Can you work these out from the model? Positions are in its coordinate system, mm. Face numbers are marked on the shaded views. A direction names the side the tool comes from. Coordinates: 2 decimals unless noted, no trailing zeros. Order: outer loops, then holes, each group sorted by start corner. A loop starts at its lowest first (then second) coordinate and runs counter-clockwise, first axis right, second up. Notation, with made-up numbers: (12.5, 52) -> (26.5, 52) arc R6 ccw to (26.5, 61) -> close; hole circle Ø11 at (15, 83.5). An arc over 180 degrees is marked (long way). Use a Markdown table: item, result. Add a question column.
1. Suppose I cut it at B-B, the plane z = 8. List the corners of the cut face in (x, y) for me, then the cut area to 3 significant figures.
2. If I drill on line 1 along Y through (x, z) = (0, 10); line 2 along Z through (x, y) = (6.75, 7.5); line 3 along Y through (x, z) = (0, -3), over which ranges is the centre line in solid material (lowest first)? Write a range as from..to.
3. Suppose I cut it at A-A, the plane y = -2. List the corners of the cut face in (x, z) for me, then the cut area to 3 significant figures.
4. For pin 1 Ø12 at (x, y) = (7.5, 8.5) entering from -Z; pin 2 Ø4 at (x, y) = (-1.5, -1) entering from -Z; pin 3 Ø4 at (y, z) = (-3.5, 15.5) entering from +X; pin 4 Ø5 at (x, z) = (-3, 11.5) entering from +Y, each with a flat end and sliding along its axis, tell me the tip position at first contact or that it passes through.
5. We'd pull the mould along Z, two halves only. Please class the marked faces 4, 5 and 6: pulls with the +Z half, pulls with the -Z half, needs draft (parallel to the pull), parting line crosses it, or undercut.
6. Suppose I cut it at C-C, the plane y = -4.5. List the corners of the cut face in (x, z) for me.
7. Suppose I cut it at D-D, the plane x = 18. List the corners of the cut face in (y, z) for me.
8. For the marked faces 1, 2 and 3, which set-ups out of +Z, -Z, +X, -X, +Y, -Y let a thin tool reach every point of the face, with its end or its side?
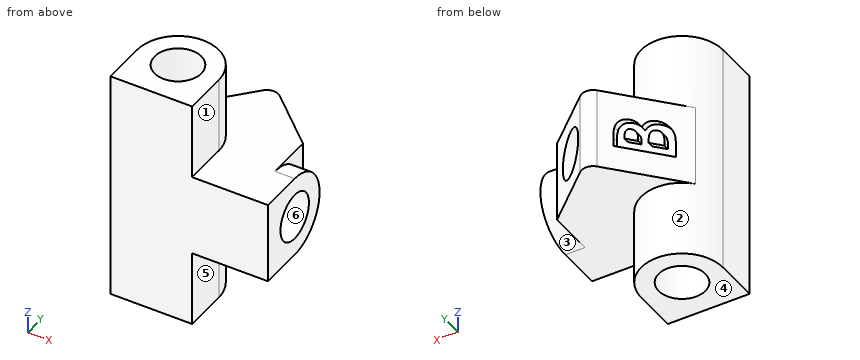
```python
from build123d import *

# Parameters (mm, degrees)
DODANIE_WYCI_GNI_CIE1_DEPTH             = 20
DODANIE_WYCI_GNI_CIE1_DEPTH_BACK        = 20
SZKIC1_R                                = 7
SZKIC1_R_2                              = 4
DODANIE_WYCI_GNI_CIE2_DEPTH             = 10
DODANIE_WYCI_GNI_CIE2_DEPTH_BACK        = 10
SZKIC2_R                                = 4
DODANIE_WYCI_GNI_CIE4_REACH             = 28.181
DODANIE_WYCI_GNI_CIE4_END_RADIUS        = 7
SZKIC3_W                                = 14
SZKIC3_H                                = 14
DODANIE_WYCI_GNI_CIE4_DIRECTION_2_DEPTH = 10
SZKIC9_R                                = 7
DODANIE_WYCI_GNI_CIE6_DEPTH             = 20
DODANIE_WYCI_GNI_CIE5_REACH             = 39.607
SZKIC12_R                               = 4
WYTNIJ_WYCI_GNI_CIE3_DEPTH              = 40.984557912
DODANIE_WYCI_GNI_CIE7_START             = 8
DODANIE_WYCI_GNI_CIE7_DEPTH             = 8.618630395
SZKIC4_R                                = 4
WYTNIJ_WYCI_GNI_CIE1_DEPTH              = 10
SZKIC10_R                               = 4
WYTNIJ_WYCI_GNI_CIE2_DEPTH              = 10
ZAOKR_GLENIE1_R                         = 2
WYTNIJ_WYCI_GNI_CIE4_DEPTH              = 1


with BuildPart() as part:
    # Szkic1 → Dodanie-wyciągnięcie1 (new, two sides: drawn at the far end of the back side and taken through both)
    with BuildSketch(Plane.XY.offset(-DODANIE_WYCI_GNI_CIE1_DEPTH_BACK)):
        Circle(SZKIC1_R)
        Circle(SZKIC1_R_2, mode=Mode.SUBTRACT)
    extrude(amount=DODANIE_WYCI_GNI_CIE1_DEPTH + DODANIE_WYCI_GNI_CIE1_DEPTH_BACK)

    # Szkic2 → Dodanie-wyciągnięcie2 (add, two sides: drawn at the far end of the back side and taken through both)
    with BuildSketch(Plane.XY.offset(-DODANIE_WYCI_GNI_CIE2_DEPTH_BACK)):
        Circle(SZKIC2_R)
    extrude(amount=DODANIE_WYCI_GNI_CIE2_DEPTH + DODANIE_WYCI_GNI_CIE2_DEPTH_BACK)

    # Dodanie-wyciągnięcie4: up to this cylinder (the profile starts outside it)
    dodanie_wyci_gni_cie4_end = Plane(origin=(0, 0, 0), z_dir=(0, 0, 1)) * Cylinder(DODANIE_WYCI_GNI_CIE4_END_RADIUS, 71.362, mode=Mode.PRIVATE)
    # Szkic3 → Dodanie-wyciągnięcie4 (add, up to the surface)
    with BuildSketch(Plane(origin=(4.711087595, 5.177417665, 0), x_dir=(0, 0, 1), z_dir=(0.6730125135097745, 0.7396310949786087, 0)), mode=Mode.PRIVATE) as dodanie_wyci_gni_cie4_sk1:
        Rectangle(SZKIC3_W, SZKIC3_H)
    dodanie_wyci_gni_cie4_tool1 = extrude(dodanie_wyci_gni_cie4_sk1.sketch, amount=-DODANIE_WYCI_GNI_CIE4_REACH, mode=Mode.PRIVATE) - dodanie_wyci_gni_cie4_end
    add(dodanie_wyci_gni_cie4_tool1.solids().sort_by_distance((4.711088, 5.177418, 0))[0])
    add(dodanie_wyci_gni_cie4_tool1.solids().sort_by_distance((4.711088, 5.177418, 0))[1])

    # Szkic3 → Dodanie-wyciągnięcie4 direction 2 (add)
    with BuildSketch(Plane(origin=(4.711087595, 5.177417665, 0), x_dir=(0, 0, 1), z_dir=(0.6730125135097745, 0.7396310949786087, 0))):
        Rectangle(SZKIC3_W, SZKIC3_H)
    extrude(amount=DODANIE_WYCI_GNI_CIE4_DIRECTION_2_DEPTH)

    # Szkic9 → Dodanie-wyciągnięcie6 (add)
    with BuildSketch(Plane(origin=(0, 0, 0), x_dir=(0, 0, -1), z_dir=(1, 0, 0))):
        Circle(SZKIC9_R)
    extrude(amount=DODANIE_WYCI_GNI_CIE6_DEPTH)

    # Szkic8 → Dodanie-wyciągnięcie5 (add, up to next)
    with BuildSketch(Plane(origin=(0, -7.5, 0), x_dir=(1, 0, 0), z_dir=(0, 1, 0)), mode=Mode.PRIVATE) as dodanie_wyci_gni_cie5_sk1:
        Polygon((7, 20), (-7, 20), (-7, -20), (7, -20), (7, -7), (20, -7), (20, 7), (7, 7), align=None)
    dodanie_wyci_gni_cie5_tool1 = extrude(dodanie_wyci_gni_cie5_sk1.sketch, amount=DODANIE_WYCI_GNI_CIE5_REACH, mode=Mode.PRIVATE) - part.part
    add(dodanie_wyci_gni_cie5_tool1.solids().sort_by_distance((3.311321, -7.5, 0))[0])

    # Szkic12 → Wytnij-wyciągnięcie3 (cut, through all)
    with BuildSketch(Plane.XY.offset(10)):
        Circle(SZKIC12_R)
    extrude(amount=-WYTNIJ_WYCI_GNI_CIE3_DEPTH, mode=Mode.SUBTRACT)

    # Dodanie-wyciągnięcie7: read off the stored shape, not the designer's step
    # Dodanie-wyciągnięcie7 outline → Dodanie-wyciągnięcie7 (add)
    with BuildSketch(Plane.YZ.offset(DODANIE_WYCI_GNI_CIE7_START)):
        with BuildLine():
            Line((7.86264102, 7), (0, 7))
            ThreePointArc((0, 7), (7, 0), (0, -7))
            Line((0, -7), (7.86264102, -7))
            Line((7.86264102, -7), (7.86264102, 7))
        make_face()
    extrude(amount=DODANIE_WYCI_GNI_CIE7_DEPTH)

    # Szkic4 → Wytnij-wyciągnięcie1 (cut)
    with BuildSketch(Plane(origin=(11.44121273, 12.573728615, 0), x_dir=(0, 0, -1), z_dir=(0.6730125135097745, 0.7396310949786088, 0))):
        with Locations(Location((0, 0, 0), (0, 0, 90))):
            Circle(SZKIC4_R)
    extrude(amount=-WYTNIJ_WYCI_GNI_CIE1_DEPTH, mode=Mode.SUBTRACT)

    # Szkic10 → Wytnij-wyciągnięcie2 (cut)
    with BuildSketch(Plane(origin=(20, 0, 0), x_dir=(0, 0, -1), z_dir=(1, 0, 0))):
        Circle(SZKIC10_R)
    extrude(amount=-WYTNIJ_WYCI_GNI_CIE2_DEPTH, mode=Mode.SUBTRACT)

    # Zaokrąglenie1
    zaokr_glenie1_edges = [part.edges().sort_by_distance(p)[0] for p in [
        (6.263795065, 17.284816209, 0),
    ]]
    fillet(zaokr_glenie1_edges, radius=ZAOKR_GLENIE1_R)

    # Szkic14 → Wytnij-wyciągnięcie4 (cut, along a direction that is not the sketch's normal)
    with BuildSketch(Plane(origin=(-5.177417665, 4.711087595, 0), x_dir=(0, 0, 1), z_dir=(-0.7396310949786086, 0.6730125135097746, 0))):
        with BuildLine():
            Line((-2.686538462, 3), (-2.686538462, 12.525))
            Line((-2.686538462, 12.525), (-1.160096154, 12.525))
            add(Edge.make_bspline(
                [(-1.160096154, 12.525), (-1.053235648, 12.525012195), (-0.846462595, 12.525035793), (-0.548143042, 12.51455979), (-0.271476851, 12.501007906), (-0.01734448, 12.4858465), (0.214686622, 12.459720367), (0.424263612, 12.432186277), (0.611805228, 12.398981861), (0.727752018, 12.369196471), (0.782301683, 12.355183293)],
                knots=[0, 0, 0, 0, 1.311965854, 2.538629056, 3.664479157, 4.713267157, 5.663616078, 6.530575999, 7.308677837, 8, 8, 8, 8], degree=3))
            add(Edge.make_bspline(
                [(0.782301683, 12.355183293), (0.85393093, 12.335417456), (0.994490509, 12.296630538), (1.195816681, 12.218298682), (1.386802639, 12.131227269), (1.567215194, 12.031895073), (1.735946541, 11.919102874), (1.892355443, 11.79195552), (2.039815254, 11.655556701), (2.173090012, 11.50610502), (2.293548434, 11.348181634), (2.398205206, 11.181827924), (2.489138527, 11.009587547), (2.561909002, 10.829292972), (2.616740188, 10.641774504), (2.656843488, 10.447832876), (2.682835858, 10.24685441), (2.685291796, 10.11012219), (2.686538462, 10.040715144)],
                knots=[0, 0, 0, 0, 1.099996261, 2.158545794, 3.195537121, 4.207578794, 5.205712374, 6.197378256, 7.190519799, 8.17788031, 9.159561366, 10.129234751, 11.085776129, 12.040971148, 13.00380137, 13.975669004, 14.972423361, 16, 16, 16, 16], degree=3))
            add(Edge.make_bspline(
                [(2.686538462, 10.040715144), (2.6832788, 9.951545308), (2.676862558, 9.776025442), (2.635875166, 9.518218515), (2.559017418, 9.274553912), (2.458450925, 9.040540989), (2.321711936, 8.817052614), (2.148079865, 8.604195051), (1.940366984, 8.395414096), (1.781039737, 8.270263996), (1.698167067, 8.205168269)],
                knots=[0, 0, 0, 0, 0.986156485, 1.941127874, 2.875419072, 3.804401753, 4.751181392, 5.761612777, 6.835722519, 8, 8, 8, 8], degree=3))
            add(Edge.make_bspline(
                [(1.698167067, 8.205168269), (1.765323103, 8.170885695), (1.89699751, 8.103667053), (2.083936483, 7.99317967), (2.257021567, 7.875662326), (2.417028822, 7.753479516), (2.560601912, 7.621451735), (2.693669212, 7.487186605), (2.809665872, 7.342991291), (2.913393581, 7.194005189), (3.00355202, 7.038070964), (3.082070078, 6.875451953), (3.148391466, 6.705592614), (3.204554132, 6.529357394), (3.246440263, 6.346140126), (3.273750912, 6.155875284), (3.294661651, 5.959211768), (3.29628831, 5.825249491), (3.297115385, 5.757136418)],
                knots=[0, 0, 0, 0, 1.164658916, 2.283573913, 3.35186032, 4.395461096, 5.390182219, 6.362969632, 7.312859996, 8.245001507, 9.165155236, 10.092416118, 11.032087915, 11.979892451, 12.947605196, 13.931445124, 14.948243989, 16, 16, 16, 16], degree=3))
            add(Edge.make_bspline(
                [(3.297115385, 5.757136418), (3.291748226, 5.627044343), (3.281156159, 5.370308155), (3.203712138, 4.993360467), (3.069448812, 4.63597987), (2.889160851, 4.299586747), (2.667011396, 3.993919126), (2.411603228, 3.726156945), (2.125507722, 3.499502202), (1.861550038, 3.346527834), (1.633247428, 3.243867728), (1.444148642, 3.180396777), (1.241060554, 3.121597384), (1.020263078, 3.080307236), (0.785758971, 3.042513952), (0.535261803, 3.019179595), (0.26923975, 3.003366477), (0.086524304, 3.001144846), (-0.007632212, 3)],
                knots=[0, 0, 0, 0, 1.284142165, 2.534249414, 3.780121997, 5.041676246, 6.291546858, 7.49970053, 8.684500223, 9.883330709, 10.50184324, 11.153274765, 11.851151195, 12.587658647, 13.369265475, 14.195992086, 15.070362669, 16, 16, 16, 16], degree=3))
            Line((-0.007632212, 3), (-2.686538462, 3))
        make_face()
        with BuildLine():
            Line((-0.976923077, 10.815384615), (-0.976923077, 8.739423077))
            Line((-0.976923077, 8.739423077), (-0.52280649, 8.739423077))
            add(Edge.make_bspline(
                [(-0.52280649, 8.739423077), (-0.461087966, 8.739961286), (-0.341944091, 8.741000265), (-0.1698534, 8.754381963), (-0.009836849, 8.77721197), (0.137498653, 8.809065573), (0.273525591, 8.849515004), (0.397374985, 8.898184382), (0.508502292, 8.957566312), (0.63760652, 9.046018318), (0.774079, 9.176179404), (0.894214189, 9.364224061), (0.964973013, 9.580474702), (0.972853637, 9.732991398), (0.976923077, 9.811748798)],
                knots=[0, 0, 0, 0, 1.065314748, 2.056525647, 2.977365736, 3.853934255, 4.656397591, 5.425096493, 6.14721249, 6.826394842, 8.123232004, 9.372140726, 10.643011755, 12, 12, 12, 12], degree=3))
            add(Edge.make_bspline(
                [(0.976923077, 9.811748798), (0.97366678, 9.885518189), (0.967370861, 10.028148341), (0.896125823, 10.228413777), (0.785468194, 10.40588994), (0.654821309, 10.527357859), (0.531791881, 10.610316867), (0.426446534, 10.664941841), (0.310822106, 10.71384156), (0.18268023, 10.751231476), (0.042752669, 10.779287553), (-0.108280873, 10.799891382), (-0.27068098, 10.813915224), (-0.382851079, 10.814884312), (-0.440760216, 10.815384615)],
                knots=[0, 0, 0, 0, 1.347982417, 2.606269829, 3.849316587, 5.153353503, 5.842674298, 6.568177932, 7.326619318, 8.142485038, 9.012069166, 9.942760135, 10.937925643, 12, 12, 12, 12], degree=3))
            Line((-0.440760216, 10.815384615), (-0.976923077, 10.815384615))
        make_face(mode=Mode.SUBTRACT)
        with BuildLine():
            Line((-0.976923077, 7.151923077), (-0.976923077, 4.709615385))
            Line((-0.976923077, 4.709615385), (-0.484645433, 4.709615385))
            add(Edge.make_bspline(
                [(-0.484645433, 4.709615385), (-0.387321516, 4.710171393), (-0.200204141, 4.711240387), (0.067841168, 4.724156384), (0.311561364, 4.747435193), (0.530310682, 4.776496911), (0.724424178, 4.815870993), (0.893245702, 4.865930091), (1.039090422, 4.921003819), (1.161083845, 4.989026413), (1.260745483, 5.068187842), (1.350679663, 5.149092725), (1.424006389, 5.242424151), (1.482023863, 5.344175661), (1.532237884, 5.451819674), (1.562523436, 5.569559649), (1.585581792, 5.693906057), (1.586850755, 5.779913778), (1.5875, 5.823918269)],
                knots=[0, 0, 0, 0, 1.753078804, 3.370512758, 4.83203934, 6.162291463, 7.344201807, 8.395507345, 9.331626367, 10.147333109, 10.898971645, 11.62040215, 12.321813352, 13.025280112, 13.727906689, 14.453419512, 15.208716525, 16, 16, 16, 16], degree=3))
            add(Edge.make_bspline(
                [(1.5875, 5.823918269), (1.586068229, 5.874238098), (1.583279523, 5.972247587), (1.560504132, 6.115498915), (1.519113807, 6.249233534), (1.466980673, 6.37687122), (1.394434648, 6.493842097), (1.308216175, 6.604194086), (1.204042251, 6.704190327), (1.086892595, 6.799878966), (0.95024912, 6.883659553), (0.794047716, 6.956354053), (0.617439814, 7.017065822), (0.41987835, 7.065404572), (0.202229419, 7.106429001), (-0.037095577, 7.130925114), (-0.296103456, 7.14914395), (-0.475703734, 7.150975652), (-0.56859976, 7.151923077)],
                knots=[0, 0, 0, 0, 0.845221588, 1.646264278, 2.427170338, 3.19324141, 3.95557735, 4.731569926, 5.540061037, 6.376114724, 7.268642756, 8.224665384, 9.265483498, 10.400594375, 11.639216012, 12.983232105, 14.439614077, 16, 16, 16, 16], degree=3))
            Line((-0.56859976, 7.151923077), (-0.976923077, 7.151923077))
        make_face(mode=Mode.SUBTRACT)
    extrude(amount=-WYTNIJ_WYCI_GNI_CIE4_DEPTH, dir=(0, 1, 0), mode=Mode.SUBTRACT)


solid = part.part
```
Worked out:
| question | item | result |
|---|---|---|
| 1 | outline | (-7, -7.5) -> (7, -7.5) -> (7, 0) arc R7 ccw to (-7, 0) -> close; hole circle Ø8 at (0, 0) |
| 1 | area | 132 mm² |
| 2 | line 1 | y = -7.5..-4, 4..7 |
| 2 | line 2 | z = -7..-4, 4..7 |
| 2 | line 3 | y = -7.5..-4, 4..10.4 |
| 3 | outline | (-7, -20) -> (-3.46, -20) -> (-3.46, 20) -> (-7, 20) -> close; (3.46, -20) -> (7, -20) -> (7, -7) -> (20, -7) -> (20, -3.46) -> (10, -3.46) -> (10, 3.46) -> (20, 3.46) -> (20, 7) -> (7, 7) -> (7, 20) -> (3.46, 20) -> close |
| 3 | area | 396 mm² |
| 4 | pin 1 | stops at z = -20 |
| 4 | pin 2 | passes through |
| 4 | pin 3 | stops at x = 7 |
| 4 | pin 4 | stops at y = 6.98 |
| 5 | face 4 | pulls with the -Z half |
| 5 | face 5 | needs draft |
| 5 | face 6 | undercut |
| 6 | outline | (-7, -20) -> (7, -20) -> (7, -7) -> (20, -7) -> (20, 7) -> (7, 7) -> (7, 20) -> (-7, 20) -> close |
| 7 | outline | (-7.5, -7) -> (0, -7) arc R7 ccw to (0, 7) -> (-7.5, 7) -> close; hole circle Ø8 at (0, 0) |
| 8 | face 1 | +Z, +X, +Y, -Y |
| 8 | face 2 | +Y |
| 8 | face 3 | +X, +Y |
